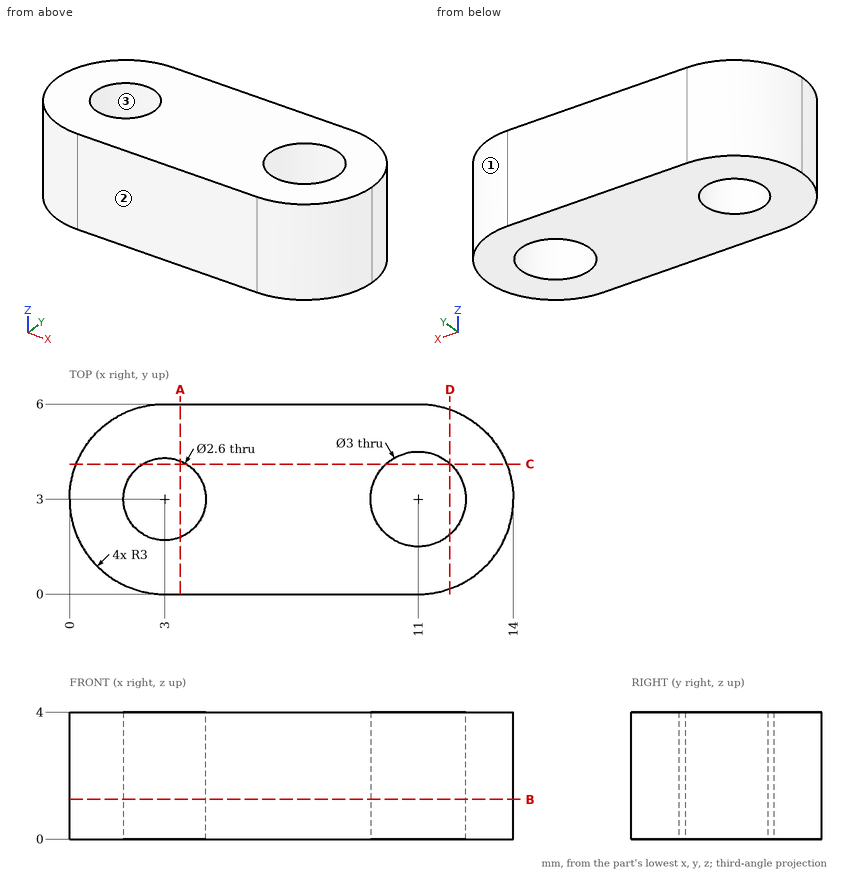
Job drawing, mm, ordinate dimensions from the low corner. One solid piece. Round coordinates to 2 decimals unless told otherwise and drop trailing zeros. Order: outer loops, then holes, each group sorted by start corner. A loop starts at its lowest first (then second) coordinate and runs counter-clockwise, first axis right, second up. Notation, with made-up numbers: (81.5, -9) -> (114.5, -9) arc R20 cw to (114.5, 14) -> close; hole circle Ø1 at (28.25, 56). An arc over 180 degrees is marked (long way). Write item = value, one per line.
(1) Cut at C-C (y = 4.1). Write the cut outline in (x, z).
Answers follow:
outline = (0.21, 0) -> (2.31, 0) -> (2.31, 4) -> (0.21, 4) -> close; (3.69, 0) -> (9.98, 0) -> (9.98, 4) -> (3.69, 4) -> close; (12.02, 0) -> (13.79, 0) -> (13.79, 4) -> (12.02, 4) -> close
(2) Cut at A-A (x = 3.5). Write the cut outline in (y, z).
Answers follow:
outline = (0, 0) -> (1.8, 0) -> (1.8, 4) -> (0, 4) -> close; (4.2, 0) -> (6, 0) -> (6, 4) -> (4.2, 4) -> close
(3) Cut at D-D (x = 12). Write the cut outline in (y, z), plus the area to 3 significant figures.
Answers follow:
outline = (0.17, 0) -> (1.88, 0) -> (1.88, 4) -> (0.17, 4) -> close; (4.12, 0) -> (5.83, 0) -> (5.83, 4) -> (4.12, 4) -> close
area = 13.7 mm²
(4) Drill centre lines: L1, parallel to X at y = 3, z = 1.4; L2, parallel to Y at x = 11, z = 3.15; L3, parallel to Y at x = 3, z = 2.55. Where is each one in solid material? Low to high.
Answers follow:
L1 = 0 to 1.7, 4.3 to 9.5, 12.5 to 14
L2 = 0 to 1.5, 4.5 to 6
L3 = 0 to 1.7, 4.3 to 6
(5) Cut at B-B (z = 1.25). State how many separate pieces and enclosed holes the cut face has, plus the area to 3 significant figures.
Answers follow:
separate_pieces = 1
enclosed_holes = 2
area = 63.9 mm²
(6) Pull direction X, two halves, no side cores. Call the marked faces 1, 2 and 3: +X half, -X half, draft (parallel to the pull), parting line (faces both ways), or undercut.
Answers follow:
face_1 = +X half
face_2 = draft
face_3 = undercut
